from build123d import *

# Parameters (mm, degrees)
RESSALTO_EXTRUS_O1_DEPTH = 10
RESSALTO_EXTRUS_O2_DEPTH = 2
ESBO_O2_W                = 5.5
ESBO_O2_H                = 8
CORTE_EXTRUS_O1_DEPTH    = 10
ESBO_O3_R                = 1.65
CORTE_EXTRUS_O2_DEPTH    = 10
ESBO_O4_R                = 2.65
CORTE_EXTRUS_O3_DEPTH    = 10
CORTE_EXTRUS_O4_START    = -1.5
CORTE_EXTRUS_O4_DEPTH    = 3
FILETE1_R                = 1


with BuildPart() as part:
    # Esboço1 → Ressalto-extrusão1 (new body)
    with BuildSketch(Plane(origin=(0, 0, 0), x_dir=(1, 0, 0), z_dir=(0, 1, 0))):
        Polygon((0, 0), (0, 20), (6, 20), (6, 5), (26.5, 5), (26.5, -20), (21.5, -20), (21.5, 0), align=None)
    extrude(amount=RESSALTO_EXTRUS_O1_DEPTH)

    # Esboço8 → Ressalto-extrusão2 (add)
    with BuildSketch(Plane.XZ):
        Polygon((26.5, -5), (6, -5), (6, -20), (0, -20), (0, 20), (26.5, 20), align=None)
    extrude(amount=RESSALTO_EXTRUS_O2_DEPTH)

    # Esboço2 → Corte-extrusão1 (cut)
    with BuildSketch(Plane.ZY.offset(-21.5)):
        with Locations((10, 4)):
            Rectangle(ESBO_O2_W, ESBO_O2_H)
    extrude(amount=-CORTE_EXTRUS_O1_DEPTH, mode=Mode.SUBTRACT)

    # Esboço3 → Corte-extrusão2 (cut)
    with BuildSketch(Plane(origin=(6, 0, 0), x_dir=(0, 0, -1), z_dir=(1, 0, 0))):
        with Locations((16.5, 3)):
            Circle(ESBO_O3_R)
    extrude(amount=-CORTE_EXTRUS_O2_DEPTH, mode=Mode.SUBTRACT)

    # Esboço4 → Corte-extrusão3 (cut)
    with BuildSketch(Plane(origin=(0, 0, -5), x_dir=(-1, 0, 0), z_dir=(0, 0, -1))):
        with Locations((-11.5, 5)):
            Circle(ESBO_O4_R)
    extrude(amount=-CORTE_EXTRUS_O3_DEPTH, mode=Mode.SUBTRACT)

    # Esboço7 → Corte-extrusão4 (cut)
    with BuildSketch(Plane.ZY.offset(CORTE_EXTRUS_O4_START)):
        Polygon((-13.035898385, 3), (-14.767949192, 6), (-18.232050808, 6), (-20, 6), (-20, 0), (-18.232050808, 0), (-14.767949192, 0), align=None)
    extrude(amount=-CORTE_EXTRUS_O4_DEPTH, mode=Mode.SUBTRACT)

    # Filete1
    filete1_edges = [part.edges().sort_by_distance(p)[0] for p in [
        (3, 10, -20),
        (21.5, 5, 20),
        (26.5, 4, 20),
        (26.5, 4, -5),
        (0, 5, 0),
        (0, -1, 20),
        (3, -2, -20),
    ]]
    fillet(filete1_edges, radius=FILETE1_R)


solid = part.part
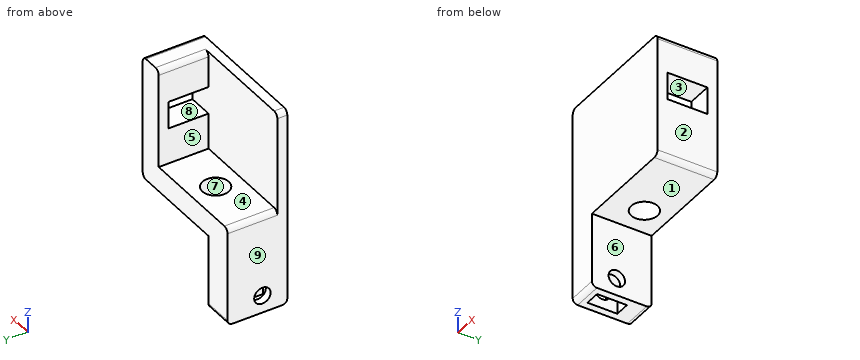
Read the model definition and answer for the solid it produces. Units are mm, in the model's axes. Face numbers are marked on the shaded views. A direction names the side the tool comes from. Round coordinates to 2 decimals unless told otherwise and drop trailing zeros. Write each loop counter-clockwise with the first axis right and the second up, starting at its lowest first coordinate (ties: lowest second). Pieces come first, ordered by that corner, then holes. Notation, with made-up numbers: (60.5, 21) - (90.5, 21) arc R26 cw to (90.5, 40) - close; hole circle Ø11 at (10, 63.25). An arc over 180 degrees is marked (long way). One line per question, with ' | ' between items. Start each with the question number.
1. Section B-B (x = 11.5) is taken. Determine the outline of the cut face in (y, z).
2. Find the intervals of material crossed by probe 1 along Y at (x, z) = (5.1, -16.5); probe 2 along Y at (x, z) = (22.25, 7.5); probe 3 along X at (y, z) = (6.25, 3), in increasing order. Write a range as [from, to].
3. Section C-C (x = 16) is taken. Determine the outline of the cut face in (y, z), and give its area (3 significant figures).
4. For a pull along Z with two mould halves and no side action, classify the marked faces 1, 2, 3 and 4 as +Z half, -Z half, draft (parallel to the pull), parting line (faces both ways), or undercut.
5. Each of these flat-tipped pins is pushed along its axis until it touches: pin 1 (8 mm diameter, centred on x = 9.5, z = 11.5, fed in from +Y); pin 2 (5.5 mm diameter, centred on y = 3, z = -16.5, fed in from +X); pin 3 (5 mm diameter, centred on y = 5.5, z = 8.5, fed in from -X). Where does it stop, or does it pass through?
6. Section D-D (z = 17) is taken. Determine the outline of the cut face in (x, y), and give its area (3 significant figures).
7. Section A-A (z = -16.5) is taken. Determine the outline of the cut face in (x, y).
8. For the marked faces 5, 6, 7, 8 and 9, determine the directions among +Z, -Z, +X, -X, +Y, -Y from which every point of the face is accessible in a straight line to the end or side of a thin tool.
Filled in:
1) outline: (-2, -5) - (2.35, -5) - (2.35, 0) - (0, 0) - (0, 20) - (-2, 20) - close; (7.65, -5) - (10, -5) - (10, 0) - (7.65, 0) - close
2) probe 1: [-2, 1.35], [4.65, 10] | probe 2: [-2, 0], [8, 10] | probe 3: [21.5, 26.5]
3) outline: (-2, -5) - (10, -5) - (10, 0) - (0, 0) - (0, 20) - (-2, 20) - close | area: 100 mm²
4) face 1: -Z half | face 2: draft | face 3: undercut | face 4: +Z half
5) pin 1: y = 0 | pin 2: x = 6 | pin 3: x = 21.5
6) outline: (0, -2) - (26.5, -2) - (26.5, 10) - (21.5, 10) - (21.5, 0) - (0, 0) - close | area: 103 mm²
7) outline: (0, -2) - (6, -2) - (6, 1.35) - (4.5, 1.35) - (4.5, 0) - (1.5, 0) - (1.5, 1.35) - (0, 1.35) - close; (0, 4.65) - (1.5, 4.65) - (1.5, 6) - (4.5, 6) - (4.5, 4.65) - (6, 4.65) - (6, 10) - (0, 10) - close
8) face 5: +Z, -X, +Y | face 6: -Z, +X, +Y, -Y | face 7: +Z, -Z | face 8: +X, -X | face 9: +Z, -Z, -X, +Y, -Y
